Input: part model. Units: mm. Frame: model coordinates. Face numbers are marked on the shaded views. Give positions to 0.01 mm unless a question says otherwise; leave off trailing zeros. Order: outer loops, then holes, each group sorted by start corner. A loop starts at its lowest first (then second) coordinate and runs counter-clockwise, first axis right, second up. Notation, with made-up numbers: M 59.5,36 L 78.5,36 A18 cw 78.5,57 Z; hole C 73,-19.75 d6. An arc over 180 degrees is marked long. Use a Markdown table: item, result.
from build123d import *

# Parameters (mm, degrees)
ESQUISSE1_R                  = 17.5
ESQUISSE1_R_2                = 15.5
BOSS_EXTRU_1_DEPTH           = 158
ENL_V_MAT_EXTRU_1_DEPTH      = 160.926545639
ENL_V_MAT_EXTRU_1_DEPTH_BACK = 160.926545639
ESQUISSE2_R                  = 2


with BuildPart() as part:
    # Esquisse1 → Boss.-Extru.1 (new body)
    with BuildSketch(Plane(origin=(0, 0, 0), x_dir=(1, 0, 0), z_dir=(0, 1, 0))):
        with Locations(Location((0, 0, 0), (0, 0, 270))):
            Circle(ESQUISSE1_R)
        with Locations(Location((0, 0, 0), (0, 0, 270))):
            Circle(ESQUISSE1_R_2, mode=Mode.SUBTRACT)
    extrude(amount=BOSS_EXTRU_1_DEPTH)

    # Esquisse2 → Enlèv. mat.-Extru.1 (cut, two sides: drawn at the far end of the back side and taken through both)
    with BuildSketch(Plane.XY.offset(-ENL_V_MAT_EXTRU_1_DEPTH_BACK)):
        with Locations((0, 146)):
            Circle(ESQUISSE2_R)
        with Locations((0, 12)):
            Circle(ESQUISSE2_R)
    extrude(amount=ENL_V_MAT_EXTRU_1_DEPTH + ENL_V_MAT_EXTRU_1_DEPTH_BACK, mode=Mode.SUBTRACT)


solid = part.part
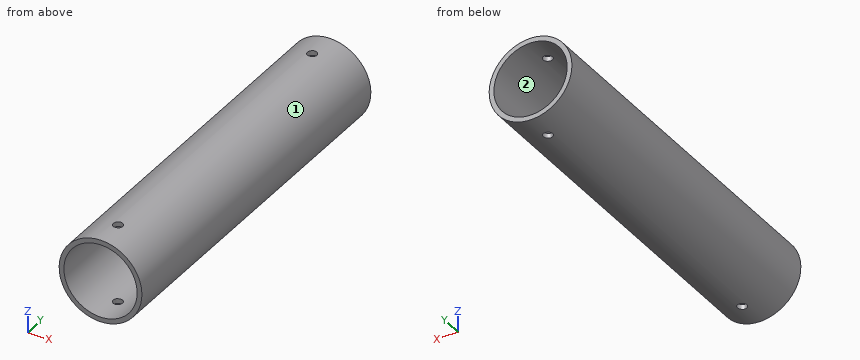
1) Mould query, pull axis X, two halves, no side actions, for the marked faces 1 and 2. Classes: released by +X, released by -X, zero draft, split by the parting line, or undercut.
Response values:
| item | result |
|---|---|
| face 1 | split by the parting line |
| face 2 | undercut |
2) Cut plane A-A on z = 0. Return loops of the section in (x, y).
Response values:
| item | result |
|---|---|
| outline | M -17.5,0 L -15.5,0 L -15.5,158 L -17.5,158 Z; M 15.5,0 L 17.5,0 L 17.5,158 L 15.5,158 Z |
3) Cut plane B-B on x = 0. Return loops of the section in (y, z), and give its area (3 significant figures).
Response values:
| item | result |
|---|---|
| outline | M 0,-17.5 L 10,-17.5 L 10,-15.5 L 0,-15.5 Z; M 0,15.5 L 10,15.5 L 10,17.5 L 0,17.5 Z; M 14,-17.5 L 144,-17.5 L 144,-15.5 L 14,-15.5 Z; M 14,15.5 L 144,15.5 L 144,17.5 L 14,17.5 Z; M 148,-17.5 L 158,-17.5 L 158,-15.5 L 148,-15.5 Z; M 148,15.5 L 158,15.5 L 158,17.5 L 148,17.5 Z |
| area | 600 mm² |
4) First-contact query: pin 1 Ø12 at (x, y) = (-7.5, 66) entering from -Z; pin 2 Ø12 at (x, z) = (-13.5, 6) entering from -Y; pin 3 Ø1 at (x, y) = (-9.5, 139) entering from -Z; pin 4 Ø10 at (x, y) = (7.5, 73) entering from -Z. Flat tips, straight axial feed; report the tip coordinate or a pass-through.
Response values:
| item | result |
|---|---|
| pin 1 | stops at z = -17.44 |
| pin 2 | stops at y = 0 |
| pin 3 | stops at z = -15.01 |
| pin 4 | stops at z = -17.32 |
5) Material intervals for line 1 (X direction, y = 55, z = 0); line 2 (X direction, y = 126, z = 7), sorted ascending. Write a range as from..to.
Response values:
| item | result |
|---|---|
| line 1 | x = -17.5..-15.5, 15.5..17.5 |
| line 2 | x = -16.04..-13.83, 13.83..16.04 |
6) Cut plane D-D on y = 96.5. Return loops of the section in (x, z), and give its area (3 significant figures).
Response values:
| item | result |
|---|---|
| outline | C 0,0 d35; hole C 0,0 d31 |
| area | 207 mm² |
